```python
from build123d import *

# Parameters (mm, degrees)
SZKIC1_R                    = 3
SZKIC1_R_2                  = 6
DODANIE_WYCI_GNI_CIE1_DEPTH = 2
SZYK_KO_OWY1_COUNT          = 4
ZAOKR_GLENIE1_DEPTH         = 2
SZKIC2_R                    = 1.55
WYTNIJ_WYCI_GNI_CIE1_DEPTH  = 30.060282321


with BuildPart() as part:
    # Szkic1 → Dodanie-wyciągnięcie1 (new body)
    with BuildSketch(Plane.XY):
        with BuildLine():
            ThreePointArc((2.400147918, 15.700197241), (-1.790710564, 15.093060932), (-2.413695775, 19.281592745))
            Line((-2.413695775, 19.281592745), (-10.062410419, 8.983603822))
            add(Edge.make_bspline(
                [(-10.062410419, 8.983603822), (-4.760498221, 10.518777319), (-8.176009399, 4.470768002), (-5.592129953, -2.174415459)],
                knots=[0, 0, 0, 0, 1, 1, 1, 1], degree=3))
            ThreePointArc((-5.592129953, -2.174415459), (-3.27017187, 5.030504541), (4.257024291, 4.228208153))
            add(Edge.make_bspline(
                [(4.257024291, 4.228208153), (0.108817482, 8.404685875), (-2.964269427, 8.546416052), (2.400147918, 15.700197241)],
                knots=[0, 0, 0, 0, 1, 1, 1, 1], degree=3))
        make_face()
        with Locations((0, 17.5)):
            Circle(SZKIC1_R)
        Circle(SZKIC1_R_2)
    dodanie_wyci_gni_cie1 = extrude(amount=DODANIE_WYCI_GNI_CIE1_DEPTH)

    # Szyk kołowy1: Dodanie-wyciągnięcie1 ×4 about axis
    szyk_ko_owy1_axis = Axis((0, 0, 0), (0, 0, -1))
    for i in range(1, SZYK_KO_OWY1_COUNT):
        add(dodanie_wyci_gni_cie1.rotate(szyk_ko_owy1_axis, i * 360 / SZYK_KO_OWY1_COUNT))

    # Zaokrąglenie1: read off the stored shape, not the designer's step
    # Zaokrąglenie1 outline → Zaokrąglenie1 (add)
    with BuildSketch(Plane.XY):
        with BuildLine():
            add(Edge.make_bspline(
                [(-6.722543952, 4.044752518), (-6.693847694, 3.317092727), (-6.646227592, 2.537215945), (-6.544838162, 1.721663177)],
                knots=[0.664728108, 0.664728108, 0.664728108, 0.664728108, 0.79801197, 0.79801197, 0.79801197, 0.79801197], degree=3))
            ThreePointArc((-6.722543952, 4.044752518), (-8.59130438, 0.500235564), (-12.595628187, 0.354438378))
            add(Edge.make_bspline(
                [(-6.544838162, 1.721663177), (-8.318139153, -0.279379709), (-9.515072999, -1.281625971), (-12.595628187, 0.354438378)],
                knots=[0.223227171, 0.223227171, 0.223227171, 0.223227171, 0.829356845, 0.829356845, 0.829356845, 0.829356845], degree=3))
        make_face()
        with BuildLine():
            add(Edge.make_bspline(
                [(-4.044752518, -6.722543952), (-3.317092725, -6.693847694), (-2.537215942, -6.646227592), (-1.721663172, -6.544838162)],
                knots=[0.664728108, 0.664728108, 0.664728108, 0.664728108, 0.79801197, 0.79801197, 0.79801197, 0.79801197], degree=3))
            ThreePointArc((-4.044752518, -6.722543952), (-0.500235564, -8.59130438), (-0.354438378, -12.595628187))
            add(Edge.make_bspline(
                [(-1.721663172, -6.544838162), (0.279379709, -8.318139153), (1.281625971, -9.515072999), (-0.354438378, -12.595628187)],
                knots=[0.223227171, 0.223227171, 0.223227171, 0.223227171, 0.829356845, 0.829356845, 0.829356845, 0.829356845], degree=3))
        make_face()
        with BuildLine():
            add(Edge.make_bspline(
                [(6.722543952, -4.044752518), (6.693847694, -3.317092727), (6.646227592, -2.537215945), (6.544838162, -1.721663177)],
                knots=[0.664728108, 0.664728108, 0.664728108, 0.664728108, 0.79801197, 0.79801197, 0.79801197, 0.79801197], degree=3))
            ThreePointArc((6.722543952, -4.044752518), (8.59130438, -0.500235564), (12.595628187, -0.354438378))
            add(Edge.make_bspline(
                [(6.544838162, -1.721663177), (8.318139153, 0.279379709), (9.515072999, 1.281625971), (12.595628187, -0.354438378)],
                knots=[0.223227171, 0.223227171, 0.223227171, 0.223227171, 0.829356845, 0.829356845, 0.829356845, 0.829356845], degree=3))
        make_face()
        with BuildLine():
            add(Edge.make_bspline(
                [(4.044752518, 6.722543952), (3.317092727, 6.693847694), (2.537215945, 6.646227592), (1.721663177, 6.544838162)],
                knots=[0.664728108, 0.664728108, 0.664728108, 0.664728108, 0.79801197, 0.79801197, 0.79801197, 0.79801197], degree=3))
            ThreePointArc((4.044752518, 6.722543952), (0.500235564, 8.59130438), (0.354438378, 12.595628187))
            add(Edge.make_bspline(
                [(1.721663177, 6.544838162), (-0.279379709, 8.318139153), (-1.281625971, 9.515072999), (0.354438378, 12.595628187)],
                knots=[0.223227171, 0.223227171, 0.223227171, 0.223227171, 0.829356845, 0.829356845, 0.829356845, 0.829356845], degree=3))
        make_face()
    extrude(amount=ZAOKR_GLENIE1_DEPTH)

    # Szkic2 → Wytnij-wyciągnięcie1 (cut, through all)
    with BuildSketch(Plane.XY.offset(2)):
        with Locations((0, 17.5)):
            Circle(SZKIC2_R)
        with Locations((17.5, 0)):
            Circle(SZKIC2_R)
        with Locations((0, -17.5)):
            Circle(SZKIC2_R)
        with Locations((-17.5, 0)):
            Circle(SZKIC2_R)
    extrude(amount=-WYTNIJ_WYCI_GNI_CIE1_DEPTH, mode=Mode.SUBTRACT)


solid = part.part
```
Build history of the part. All positions in model axes, mm. A direction names the side the tool comes from. Round coordinates to 2 decimals unless told otherwise and drop trailing zeros. Write each loop counter-clockwise with the first axis right and the second up, starting at its lowest first coordinate (ties: lowest second). Pieces come first, ordered by that corner, then holes. Notation, with made-up numbers: (81.25, -12.5) - (133.25, -12.5) arc R24 cw to (133.25, 19.5) - close; hole circle Ø6 at (26.5, -32.75). An arc over 180 degrees is marked (long way). Write each question's results on one line, items separated by ' | '. Start each with the question number.
Item 1: Saw through at B-B (y = -17.5). Write the cut outline in (x, z).
Item 2: Which spindle directions (+Z, -Z, +X, -X, +Y, -Y) get a long thin tool onto all of the face, cutting with end or side? Do faces 4 (the face through (-8.542, 0.532, 0.986)), 5 (the face through (6.185, -14.205, 0.986)). Say none if no direction does.
Item 3: Mould opens along X. For faces 1 (the face through (1.8, 19.9, 1)), 2 (the face through (0.532, 8.542, 0.986)), 3 (the face through (-6.185, 14.205, 0.986)) say: pulls with the +X half, pulls with the -X half, needs draft (parallel to the pull), parting line crosses it, or undercut.
Item 4: Wall check: L1, parallel to X at y = 1, z = 0.2; L2, parallel to Y at x = -17.5, z = 0.6; L3, parallel to X at y = -2.5, z = 1.95. Give the ranges that are in metal, low to high. Write a range as [from, to].
Item 5: Saw through at A-A (x = -17). Write the cut outline in (y, z), and give its area (3 significant figures).
Item 6: Drop a flat-ended pin along its axis: P1, Ø3, axis at x = 17.5, y = 0, coming from the +Z side. Give the stop position or say it passes through.
Item 7: Saw through at C-C (z = 1.1). State how many separate pieces and enclosed holes the cut face has, and give its area (3 significant figures).
Results are:
1) outline: (-3, 0) - (-1.55, 0) - (-1.55, 2) - (-3, 2) - close; (1.55, 0) - (3.74, 0) - (3.74, 2) - (1.55, 2) - close
2) face 4: +Z, -Z | face 5: +Z, -Z, +X, -Y
3) face 1: parting line crosses it | face 2: undercut | face 3: pulls with the -X half
4) L1: x = [-20.33, -18.68], [-16.32, -13.7], [-7.95, 16.32], [18.68, 20.33] | L2: y = [-3.74, -1.55], [1.55, 3] | L3: x = [-19.17, 6.97], [15.84, 19.16]
5) outline: (-4.11, 0) - (-1.47, 0) - (-1.47, 2) - (-4.11, 2) - close; (1.47, 0) - (2.96, 0) - (2.96, 2) - (1.47, 2) - close | area: 8.26 mm²
6) P1: passes through
7) separate pieces: 1 | enclosed holes: 4 | area: 556 mm²
